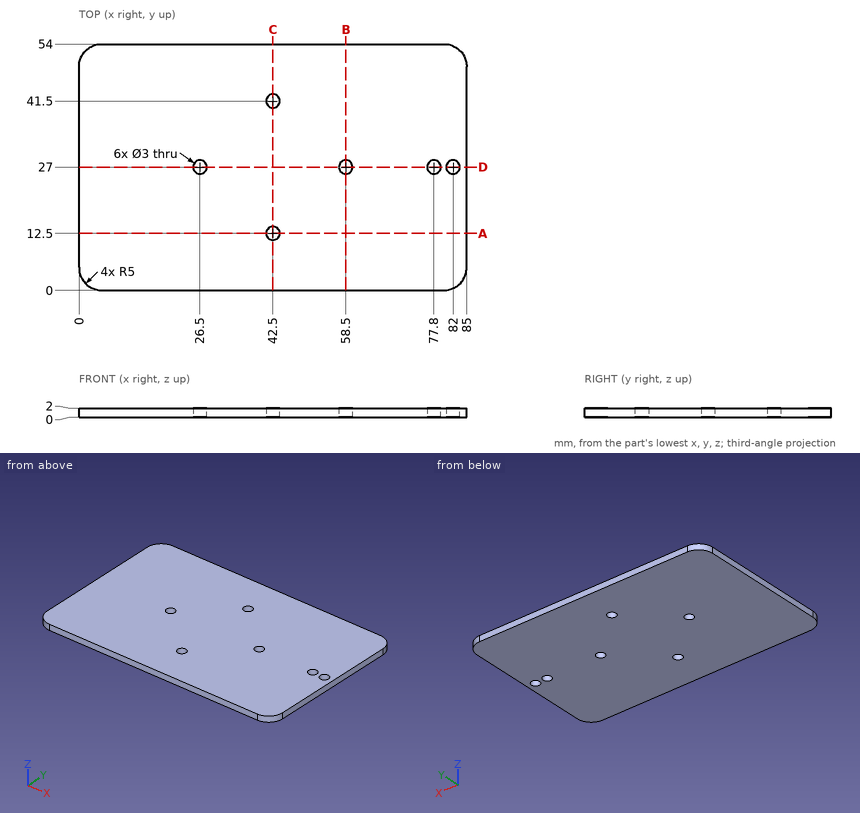
Geometry check sheet. Reference: drawing and pictorial views, mm from the part's lowest x, y, z. Round coordinates to 2 decimals unless told otherwise and drop trailing zeros. Loops run counter-clockwise (first coordinate to the right, second up) from the corner with the lowest first, then second, coordinate; pieces in that order, holes last. Notation, with made-up numbers: (-4, 81.5) - (39, 81.5) arc R20 cw to (39, 106.5) - close; hole circle Ø4 at (67, 51). An arc over 180 degrees is marked (long way). One line per question, with ' | ' between items. Start each with the question number.
1. Cross-section at C-C on x = 42.5. Record the cut outline in (y, z), then the cut area to 3 significant figures.
2. Depth check by flat-ended pin: pin 1 (2.5 mm diameter, centred on x = 82, y = 27, fed in from -Z). Enter the tip coordinate at first touch or a pass-through.
3. Scan lines: line 1 (Y direction, x = 42.5, z = 1.4); line 2 (Y direction, x = 26.5, z = 0.55); line 3 (Y direction, x = 82, z = 0.4). Record each from-to range of solid material in increasing order. Write a range as [from, to].
4. Cross-section at D-D on y = 27. Record the cut outline in (x, z).
5. Cross-section at A-A on y = 12.5. Record the cut outline in (x, z), then the cut area to 3 significant figures.
6. Cross-section at B-B on x = 58.5. Record the cut outline in (y, z).
Taken from the geometry:
1) outline: (0, 0) - (11, 0) - (11, 2) - (0, 2) - close; (14, 0) - (40, 0) - (40, 2) - (14, 2) - close; (43, 0) - (54, 0) - (54, 2) - (43, 2) - close | area: 96.0 mm²
2) pin 1: through
3) line 1: [0, 11], [14, 40], [43, 54] | line 2: [0, 25.5], [28.5, 54] | line 3: [0.42, 25.5], [28.5, 53.58]
4) outline: (0, 0) - (25, 0) - (25, 2) - (0, 2) - close; (28, 0) - (57, 0) - (57, 2) - (28, 2) - close; (60, 0) - (76.3, 0) - (76.3, 2) - (60, 2) - close; (79.3, 0) - (80.5, 0) - (80.5, 2) - (79.3, 2) - close; (83.5, 0) - (85, 0) - (85, 2) - (83.5, 2) - close
5) outline: (0, 0) - (41, 0) - (41, 2) - (0, 2) - close; (44, 0) - (85, 0) - (85, 2) - (44, 2) - close | area: 164 mm²
6) outline: (0, 0) - (25.5, 0) - (25.5, 2) - (0, 2) - close; (28.5, 0) - (54, 0) - (54, 2) - (28.5, 2) - close
